Source: CAD feature listing. Evaluate the final solid. Frame: model axes, mm. Coordinates: 2 decimals unless noted, no trailing zeros. Write each loop counter-clockwise with the first axis right and the second up, starting at its lowest first coordinate (ties: lowest second). Pieces come first, ordered by that corner, then holes. Notation, with made-up numbers: M -18,27 L -3,27 A25 cw -3,51 Z; hole C -15.75,-21.75 d8. An arc over 180 degrees is marked long. One line per item, written item: value. Start each with the question number.
Item 1: Cut plane A-A, the plane y = 0. Output: boundary loops of the cut face in (x, z), then the cut area to 3 significant figures.
Item 2: Mould query, pull axis Y, two halves, no side actions, for faces 1 (the flat face through (-1, -19, 30)), 2 (the cylindrical face through (-0.867, -3.905, 14.79)), 3 (the cylindrical face through (95.38, 30.04, 14.93)). Classes: released by +Y, released by -Y, zero draft, split by the parting line, or undercut.
Item 3: Pin query (flat end, axial travel): P1, Ø10, axis at x = 50, z = 12, coming from the -Y side; P2, Ø1, axis at y = -59, z = 24, coming from the +X side; P3, Ø6, axis at x = 68, z = 9, coming from the -Y side. Return the tip coordinate at first contact, or that it passes through.
Item 4: Ray query, L1, parallel to Y at x = 0, z = 15.75; L2, parallel to Y at x = -28.5, z = 18; L3, parallel to X at y = 72, z = 6.75. Return the intervals inside material, ascending. Write a range as from..to.
Item 5: Cut plane C-C, the plane z = 17. Output: boundary loops of the cut face in (x, y), then the cut area to 3 significant figures.
```python
from build123d import *

# Parameters (mm, degrees)
CROQUIS1_R              = 100
CROQUIS1_R_2            = 4
SALIENTE_EXTRUIR1_DEPTH = 30
REDONDEO1_R             = 10
REDONDEO2_R             = 10


with BuildPart() as part:
    # Croquis1 → Saliente-Extruir1 (new body)
    with BuildSketch(Plane.XY):
        Circle(CROQUIS1_R)
        Circle(CROQUIS1_R_2, mode=Mode.SUBTRACT)
    extrude(amount=SALIENTE_EXTRUIR1_DEPTH)

    # Redondeo1
    redondeo1_edges = [part.edges().sort_by_distance(p)[0] for p in [
        (-100, 0, 30),
    ]]
    fillet(redondeo1_edges, radius=REDONDEO1_R)

    # Redondeo2
    redondeo2_edges = [part.edges().sort_by_distance(p)[0] for p in [
        (-100, 0, 0),
    ]]
    fillet(redondeo2_edges, radius=REDONDEO2_R)


solid = part.part
```
From the geometry:
1. outline: M -100,10 A10 ccw -90,0 L -4,0 L -4,30 L -90,30 A10 ccw -100,20 Z; M 4,0 L 90,0 A10 ccw 100,10 L 100,20 A10 ccw 90,30 L 4,30 Z
1. area: 5,670 mm²
2. face 1: zero draft
2. face 2: undercut
2. face 3: split by the parting line
3. P1: stops at y = -89.3
3. P2: stops at x = 80.15
3. P3: stops at y = -75.95
4. L1: y = -100..-4, 4..100
4. L2: y = -95.85..95.85
4. L3: x = -68.61..68.61
5. outline: C 0,0 d200; hole C 0,0 d8
5. area: 31,400 mm²
